from build123d import *

# Parameters (mm, degrees)
PAD_DEPTH       = 15
SKETCH001_R     = 2.1
POCKET_DEPTH    = 54.001
SKETCH002_R     = 3.55
POCKET001_DEPTH = 4


with BuildPart() as part:
    # Sketch → Pad (new body)
    with BuildSketch(Plane.XY):
        with BuildLine():
            Line((-25, 12), (25, 12))
            Line((25, 12), (25, 32))
            Line((25, 32), (29, 32))
            Line((29, 32), (29, 3.998833))
            ThreePointArc((25.001167, 0), (27.828769, 1.171231), (29, 3.998833))
            Line((25.001167, 0), (-24.998833, 0))
            ThreePointArc((-29, 4.001167), (-27.828085, 1.171915), (-24.998833, 0))
            Line((-29, 4.001167), (-29, 54))
            Line((-29, 54), (-25, 54))
            Line((-25, 54), (-25, 12))
        make_face()
    extrude(amount=PAD_DEPTH)

    # Sketch001 → Pocket (cut, through all)
    with BuildSketch(Plane.XZ):
        with Locations((18, 7.5)):
            Circle(SKETCH001_R)
    extrude(amount=-POCKET_DEPTH, mode=Mode.SUBTRACT)

    # Sketch002 → Pocket001 (cut)
    with BuildSketch(Plane(origin=(0, 12, 0), x_dir=(-1, 0, 0), z_dir=(0, 1, 0))):
        with Locations((-18, 7.5)):
            Circle(SKETCH002_R)
    extrude(amount=-POCKET001_DEPTH, mode=Mode.SUBTRACT)


solid = part.part
Source: CAD feature listing. Evaluate the final solid. Frame: model axes, mm. A direction names the side the tool comes from. Coordinates: 2 decimals unless noted, no trailing zeros. Loops run counter-clockwise (first coordinate to the right, second up) from the corner with the lowest first, then second, coordinate; pieces in that order, holes last. Notation, with made-up numbers: (26, 34.25) - (75, 34.25) arc R10 cw to (75, 45.25) - close; hole circle Ø1 at (-3.75, -36.75). An arc over 180 degrees is marked (long way). One line per item, written item: value. Start each with the question number.
1. Section A-A (z = 7.5). Return the cut outline in (x, y).
2. Contact query for flat-ended pins moving along their axis: P1, Ø3, axis at y = 37, z = 5.5, coming from the +X side; P2, Ø3, axis at x = -18.5, z = 10.5, coming from the +Y side; P3, Ø3, axis at x = 27, z = 4.5, coming from the +Y side. Output: stop coordinate, or through.
3. Section D-D (z = 2). Return the cut outline in (x, y).
4. Ray query, L1, parallel to Z at x = 18, y = 10.5; L2, parallel to X at y = 25, z = 11; L3, parallel to Y at x = -8, z = 6.25. Return the intervals inside material, ascending.
5. Set-up query: faces 5 (the flat face through (27, 32, 7)), 6 (the flat face through (-25, 33, 7)), 7 (the flat face through (16, 8, 6)). Return all of +Z, -Z, +X, -X, +Y, -Y with unobstructed straight access to the full face (end or side cutting, diameter ignored); none if empty.
6. Section C-C (y = 15.5). Return the cut outline in (x, z), and give its area (3 significant figures).
7. Section B-B (x = 18). Return the cut outline in (y, z), and give its area (3 significant figures).
8. Mould query, pull axis Z, two halves, no side actions, for faces 1 (the flat face through (29, 18, 7)), 2 (the flat face through (-4, 11, 15)), 3 (the cylindrical face through (16.36, 10.03, 4.35)), 4 (the cylindrical face through (19.13, 3.94, 9.27)). Classes: pulls with the +Z half, pulls with the -Z half, needs draft (parallel to the pull), parting line crosses it, or undercut.
Verdict:
1. outline: (-29, 4) arc R4 ccw to (-25, 0) - (15.9, 0) - (15.9, 8) - (14.45, 8) - (14.45, 12) - (-25, 12) - (-25, 54) - (-29, 54) - close; (20.1, 0) - (25, 0) arc R4 ccw to (29, 4) - (29, 32) - (25, 32) - (25, 12) - (21.55, 12) - (21.55, 8) - (20.1, 8) - close
2. P1: stops at x = -25
2. P2: stops at y = 12
2. P3: stops at y = 32
3. outline: (-29, 4) arc R4 ccw to (-25, 0) - (25, 0) arc R4 ccw to (29, 4) - (29, 32) - (25, 32) - (25, 12) - (-25, 12) - (-25, 54) - (-29, 54) - close
4. L1: z = 0 to 3.95, 11.05 to 15
4. L2: x = -29 to -25, 25 to 29
4. L3: y = 0 to 12
5. face 5: +Z, -Z, +X, +Y
5. face 6: +Z, -Z, +Y
5. face 7: +Y
6. outline: (-29, 0) - (-25, 0) - (-25, 15) - (-29, 15) - close; (25, 0) - (29, 0) - (29, 15) - (25, 15) - close
6. area: 120 mm2
7. outline: (0, 0) - (12, 0) - (12, 3.95) - (8, 3.95) - (8, 5.4) - (0, 5.4) - close; (0, 9.6) - (8, 9.6) - (8, 11.05) - (12, 11.05) - (12, 15) - (0, 15) - close
7. area: 118 mm2
8. face 1: needs draft
8. face 2: pulls with the +Z half
8. face 3: undercut
8. face 4: undercut
